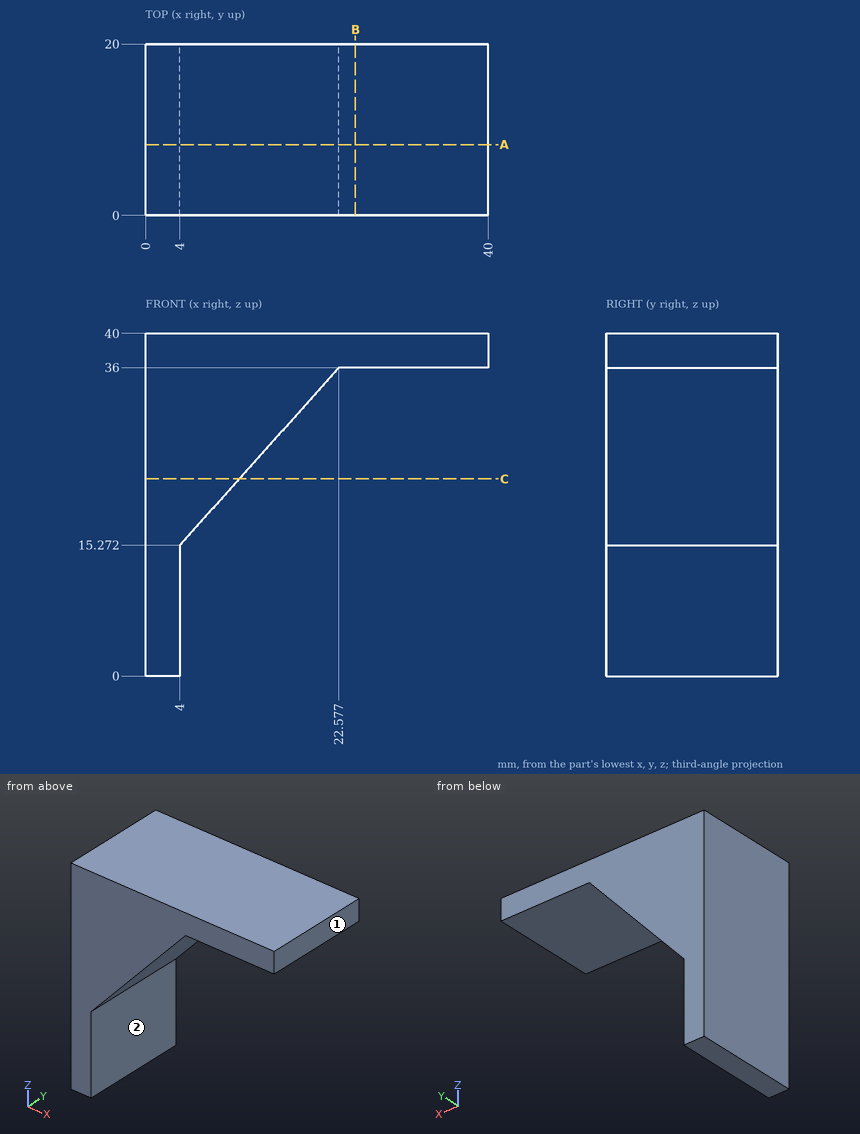
Part print with two shaded views. Sizes in mm from the minimum x, y, z corner. A direction names the side the tool comes from. Round coordinates to 2 decimals unless told otherwise and drop trailing zeros. Order: outer loops, then holes, each group sorted by start corner. A loop starts at its lowest first (then second) coordinate and runs counter-clockwise, first axis right, second up. Notation, with made-up numbers: (20, 35.25) - (65, 35.25) arc R19 ccw to (65, 48.25) - close; hole circle Ø9 at (-36, 77.5). An arc over 180 degrees is marked (long way). Answer in a Markdown table with one row per item. Add a question column.
(1) Band-saw the part on A-A on y = 8.25. List the corners of the cut face in (x, z).
(2) Probe L1, parallel to Z at x = 26, y = 19; L2, parallel to X at y = 12.5, z = 4; L3, parallel to Z at x = 15.5, y = 15 (1 decimal). List the from-to ranges inside material, lowest first. Write a range as [from, to].
(3) Band-saw the part on C-C on z = 23. List the corners of the cut face in (x, y).
(4) Band-saw the part on B-B on x = 24.5. List the corners of the cut face in (y, z), and give its area (3 significant figures).
(5) Drop flat-ended pins along their axis: pin 1 Ø8.5 at (x, y) = (27.5, 6) entering from -Z; pin 2 Ø1.5 at (y, z) = (7, 18) entering from +X; pin 3 Ø5 at (y, z) = (14.5, 24.5) entering from +X. Give the stop position or say it passes through.
(6) 3-axis set-ups, long thin cutter, end or side, ignore diameter. For the marked faces 1 and 2: which of +Z, -Z, +X, -X, +Y, -Y reach the whole face in a straight line?
Data:
| question | item | result |
|---|---|---|
| 1 | outline | (0, 0) - (4, 0) - (4, 15.27) - (22.58, 36) - (40, 36) - (40, 40) - (0, 40) - close |
| 2 | L1 | z = [36, 40] |
| 2 | L2 | x = [0, 4] |
| 2 | L3 | z = [28.1, 40] |
| 3 | outline | (0, 0) - (10.93, 0) - (10.93, 20) - (0, 20) - close |
| 4 | outline | (0, 36) - (20, 36) - (20, 40) - (0, 40) - close |
| 4 | area | 80.0 mm^2 |
| 5 | pin 1 | stops at z = 36 |
| 5 | pin 2 | stops at x = 7.12 |
| 5 | pin 3 | stops at x = 14.51 |
| 6 | face 1 | +Z, -Z, +X, +Y, -Y |
| 6 | face 2 | -Z, +X, +Y, -Y |
